```python
from build123d import *

# Parameters (mm, degrees)
SKETCH_1_W          = 140
SKETCH_1_H          = 110
SKETCH_1_R          = 41.75
EXTRUDE_2_DEPTH     = 20
SKETCH_3_R          = 46
SKETCH_3_R_2        = 41.75
EXTRUDE_3_DEPTH     = 60
SKETCH_4_W          = 21
SKETCH_4_H          = 21
CUT_EXTRUDE_1_DEPTH = 81
SKETCH_6_W          = 9
SKETCH_6_H          = 8
EXTRUDE_4_DEPTH     = 2
SKETCH_7_W          = 9
SKETCH_7_H          = 8
EXTRUDE_5_DEPTH     = 2
CUT_EXTRUDE_2_REACH = 112
SKETCH_8_W          = 40
SKETCH_8_H          = 20


with BuildPart() as part:
    # 草圖1 → 填料-伸長2 (new body)
    with BuildSketch(Plane.XY):
        Rectangle(SKETCH_1_W, SKETCH_1_H)
        Circle(SKETCH_1_R, mode=Mode.SUBTRACT)
    extrude(amount=EXTRUDE_2_DEPTH)

    # 草圖3 → 填料-伸長3 (add)
    with BuildSketch(Plane.XY.offset(20)):
        Circle(SKETCH_3_R)
        Circle(SKETCH_3_R_2, mode=Mode.SUBTRACT)
    extrude(amount=EXTRUDE_3_DEPTH)

    # 草圖4 → 除料-伸長1 (cut, through all)
    with BuildSketch(Plane(origin=(0, 0, 0), x_dir=(-1, 0, 0), z_dir=(0, 0, -1))):
        with Locations((53.5, 0.5)):
            Rectangle(SKETCH_4_W, SKETCH_4_H)
        with Locations((-53.5, 0.5)):
            Rectangle(SKETCH_4_W, SKETCH_4_H)
    extrude(amount=-CUT_EXTRUDE_1_DEPTH, mode=Mode.SUBTRACT)

    # 草圖6 → 填料-伸長4 (add)
    with BuildSketch(Plane(origin=(-41.75, 0, 0), x_dir=(0, 0, -1), z_dir=(1, 0, 0))):
        with Locations((-67.5, 0.5)):
            Rectangle(SKETCH_6_W, SKETCH_6_H)
    extrude(amount=EXTRUDE_4_DEPTH)

    # 草圖7 → 填料-伸長5 (add)
    with BuildSketch(Plane.ZY.offset(-41.75)):
        with Locations((67.5, 0.5)):
            Rectangle(SKETCH_7_W, SKETCH_7_H)
    extrude(amount=EXTRUDE_5_DEPTH)

    # 草圖8 → 除料-伸長2 (cut, up to next)
    with BuildSketch(Plane(origin=(0, 55, 0), x_dir=(1, 0, 0), z_dir=(0, 1, 0)), mode=Mode.PRIVATE) as cut_extrude_2_sk1:
        with Locations((0, -10)):
            Rectangle(SKETCH_8_W, SKETCH_8_H)
    cut_extrude_2_tool1 = extrude(cut_extrude_2_sk1.sketch, amount=-CUT_EXTRUDE_2_REACH, mode=Mode.PRIVATE) & part.part
    add(cut_extrude_2_tool1.solids().sort_by_distance((0, 55, 10))[0], mode=Mode.SUBTRACT)


solid = part.part
```
Input: part model. Units: mm. Frame: model coordinates. A direction names the side the tool comes from. Round coordinates to 2 decimals unless told otherwise and drop trailing zeros. Loops run counter-clockwise (first coordinate to the right, second up) from the corner with the lowest first, then second, coordinate; pieces in that order, holes last. Notation, with made-up numbers: (67.25, 84.5) -> (91.25, 84.5) arc R6 cw to (91.25, 93.5) -> close; hole circle Ø8 at (58.25, 6). An arc over 180 degrees is marked (long way). Use one line per item in the form item = value. Start each with the question number.
Item 1: Section query C-C on z = 53. Return the cut outline in (x, y).
Item 2: Mould query, pull axis X, two halves, no side actions, for faces 1 (the face through (19.265, -37.039, 39.44)), 2 (the face through (-45, 55, 10)), 3 (the face through (0.86, 45.99, 49.58)), 4 (the face through (39.75, 1, 67)). Classes: pulls with the +X half, pulls with the -X half, needs draft (parallel to the pull), parting line crosses it, or undercut.
Item 3: Section query B-B on x = 0. Return the cut outline in (y, z).
Item 4: Material intervals for L1, parallel to X at y = 0, z = 16; L2, parallel to Y at x = 0, z = 29.5; L3, parallel to X at y = 0, z = 53.5, sorted ascending. Write a range as from..to.
Item 5: Set-up query: faces 5 (the face through (-70, -1, 10)), 6 (the face through (-0.87, -45.99, 49.58)), 7 (the face through (-20, 46, 10)), 8 (the face through (45, 55, 10)), 9 (the face through (-52, 11, 19)). Return all of +Z, -Z, +X, -X, +Y, -Y with unobstructed straight access to the full face (end or side cutting, diameter ignored); none if empty.
Item 6: Section query A-A on y = 0. Return the cut outline in (x, z), then the cut area to 3 significant figures.
Item 7: Section query D-D on y = -32.5. Return the cut outline in (x, z), then the cut area to 3 significant figures.
Item 8: Contact query for flat-ended pins moving along their axis: pin 1 Ø1 at (x, y) = (41, 2) entering from +Z; pin 2 Ø1 at (y, z) = (-4, 46) entering from +X; pin 3 Ø2 at (y, z) = (-43.5, 38) entering from -X; pin 4 Ø17 at (x, z) = (55.5, 40) entering from -Y. Output: stop coordinate, or through.
Ans:
q1.outline = (-44.9, -10) arc R46 ccw to (44.9, -10) -> (43, -10) -> (43, 11) -> (44.67, 11) arc R46 ccw to (-44.67, 11) -> (-43, 11) -> (-43, -10) -> close; hole circle Ø83.5 at (0, 0)
q2.face_1 = undercut
q2.face_2 = needs draft
q2.face_3 = parting line crosses it
q2.face_4 = undercut
q3.outline = (-55, 0) -> (-41.75, 0) -> (-41.75, 80) -> (-46, 80) -> (-46, 20) -> (-55, 20) -> close; (41.75, 20) -> (46, 20) -> (46, 80) -> (41.75, 80) -> close
q4.L1 = -70..-64, -43..-41.75, 41.75..43, 64..70
q4.L2 = -46..-41.75, 41.75..46
q4.L3 = -43..-41.75, 41.75..43
q5.face_5 = +Z, -Z, -X, +Y, -Y
q5.face_6 = +Z, -Y
q5.face_7 = -Z, +Y
q5.face_8 = +Z, -Z, +X, -X, +Y
q5.face_9 = +Z, -Z
q6.outline = (-70, 0) -> (-64, 0) -> (-64, 20) -> (-70, 20) -> close; (-43, 0) -> (-41.75, 0) -> (-41.75, 63) -> (-39.75, 63) -> (-39.75, 72) -> (-41.75, 72) -> (-41.75, 80) -> (-43, 80) -> close; (39.75, 63) -> (41.75, 63) -> (41.75, 0) -> (43, 0) -> (43, 80) -> (41.75, 80) -> (41.75, 72) -> (39.75, 72) -> close; (64, 0) -> (70, 0) -> (70, 20) -> (64, 20) -> close
q6.area = 476 mm^2
q7.outline = (-70, 0) -> (-26.21, 0) -> (-26.21, 80) -> (-32.55, 80) -> (-32.55, 20) -> (-70, 20) -> close; (26.21, 0) -> (70, 0) -> (70, 20) -> (32.55, 20) -> (32.55, 80) -> (26.21, 80) -> close
q7.area = 2,510 mm^2
q8.pin_1 = 72
q8.pin_2 = 43
q8.pin_3 = -17.6
q8.pin_4 = through
